```python
from build123d import *
from OCP.BRepFilletAPI import BRepFilletAPI_MakeChamfer

# Parameters (mm, degrees)
SKETCH1_W               = 27
SKETCH1_H               = 32.5
BOSS_EXTRUDE1_DEPTH     = 30
SKETCH2_W               = 14
SKETCH2_H               = 18.95
BOSS_EXTRUDE2_DEPTH     = 42.5
SKETCH3_W               = 6
SKETCH3_H               = 10
CUT_EXTRUDE1_DEPTH      = 16
FILLET1_R               = 1.49
CUT_EXTRUDE2_DEPTH      = 70.576863971
CUT_EXTRUDE2_DEPTH_BACK = 70.576863971
SKETCH4_R               = 2.1
CHAMFER1_SIZE           = 3
CHAMFER1_SIZE2          = 1.732050808
SKETCH5_W               = 5
SKETCH5_H               = 18.95
BOSS_EXTRUDE3_DEPTH     = 59
FILLET2_R               = 2


with BuildPart() as part:
    # Sketch1 → Boss-Extrude1 (new, symmetric)
    with BuildSketch(Plane.XY):
        with BuildLine():
            Line((14.75, -16.3), (14.75, 16.3))
            ThreePointArc((14.75, 16.3), (14.398528137, 17.148528137), (13.55, 17.5))
            Line((13.55, 17.5), (-13.55, 17.5))
            ThreePointArc((-13.55, 17.5), (-14.398528137, 17.148528137), (-14.75, 16.3))
            Line((-14.75, 16.3), (-14.75, -16.3))
            ThreePointArc((-14.75, -16.3), (-14.398528137, -17.148528137), (-13.55, -17.5))
            Line((-13.55, -17.5), (13.55, -17.5))
            ThreePointArc((13.55, -17.5), (14.398528137, -17.148528137), (14.75, -16.3))
        make_face()
        Rectangle(SKETCH1_W, SKETCH1_H, mode=Mode.SUBTRACT)
    extrude(amount=BOSS_EXTRUDE1_DEPTH, both=True)

    # Sketch2 → Boss-Extrude2 (add, symmetric)
    with BuildSketch(Plane(origin=(0, 0, 0), x_dir=(0, 0, -1), z_dir=(1, 0, 0))):
        with Locations((-36.5, -25.775)):
            Rectangle(SKETCH2_W, SKETCH2_H)
        with Locations((36.5, -25.775)):
            Rectangle(SKETCH2_W, SKETCH2_H)
    extrude(amount=BOSS_EXTRUDE2_DEPTH, both=True)

    # Sketch3 → Cut-Extrude1 (cut)
    with BuildSketch(Plane.XZ.offset(35.25)):
        with Locations((-27, 34.5)):
            Rectangle(SKETCH3_W, SKETCH3_H)
        with Locations((-9, 34.5)):
            Rectangle(SKETCH3_W, SKETCH3_H)
        with Locations((27, 34.5)):
            Rectangle(SKETCH3_W, SKETCH3_H)
        with Locations((9, 34.5)):
            Rectangle(SKETCH3_W, SKETCH3_H)
        with Locations((9, -34.5)):
            Rectangle(SKETCH3_W, SKETCH3_H)
        with Locations((27, -34.5)):
            Rectangle(SKETCH3_W, SKETCH3_H)
        with Locations((-9, -34.5)):
            Rectangle(SKETCH3_W, SKETCH3_H)
        with Locations((-27, -34.5)):
            Rectangle(SKETCH3_W, SKETCH3_H)
    extrude(amount=-CUT_EXTRUDE1_DEPTH, mode=Mode.SUBTRACT)

    # Fillet1
    fillet1_edges = [part.edges().sort_by_distance(p)[0] for p in [
        (6, -27.25, -39.5),
        (12, -27.25, 39.5),
        (12, -27.25, 29.5),
        (6, -27.25, 29.5),
        (6, -27.25, 39.5),
        (30, -27.25, 39.5),
        (30, -27.25, 29.5),
        (24, -27.25, 29.5),
        (24, -27.25, 39.5),
        (-12, -27.25, 29.5),
        (-12, -27.25, 39.5),
        (-6, -27.25, 39.5),
        (-6, -27.25, 29.5),
        (24, -27.25, -29.5),
        (30, -27.25, -29.5),
        (30, -27.25, -39.5),
        (24, -27.25, -39.5),
        (-12, -27.25, -29.5),
        (-6, -27.25, -29.5),
        (-6, -27.25, -39.5),
        (-12, -27.25, -39.5),
        (-30, -27.25, -29.5),
        (-24, -27.25, -29.5),
        (-24, -27.25, -39.5),
        (-30, -27.25, -39.5),
        (-30, -27.25, 29.5),
        (-30, -27.25, 39.5),
        (-24, -27.25, 39.5),
        (-24, -27.25, 29.5),
        (-42.5, -25.775, 29.5),
        (-42.5, -25.775, 43.5),
        (42.5, -25.775, 29.5),
        (42.5, -25.775, 43.5),
        (-42.5, -25.775, -29.5),
        (-42.5, -25.775, -43.5),
        (42.5, -25.775, -29.5),
        (42.5, -25.775, -43.5),
        (6, -27.25, -29.5),
        (12, -27.25, -29.5),
        (12, -27.25, -39.5),
    ]]
    fillet(fillet1_edges, radius=FILLET1_R)

    # Sketch4 → Cut-Extrude2 (cut, two sides: drawn at the far end of the back side and taken through both)
    with BuildSketch(Plane(origin=(0, -16.3, 0), x_dir=(1, 0, 0), z_dir=(0, 1, 0)).offset(-CUT_EXTRUDE2_DEPTH_BACK)):
        with Locations(Location((36.25, -36.25, 0), (0, 0, 270))):
            Circle(SKETCH4_R)
        with Locations(Location((-36.25, -36.25, 0), (0, 0, 90))):
            Circle(SKETCH4_R)
        with Locations(Location((-36.25, 36.25, 0), (0, 0, 270))):
            Circle(SKETCH4_R)
        with Locations(Location((36.25, 36.25, 0), (0, 0, 90))):
            Circle(SKETCH4_R)
    extrude(amount=CUT_EXTRUDE2_DEPTH + CUT_EXTRUDE2_DEPTH_BACK, mode=Mode.SUBTRACT)

    # Chamfer1: one chamfer whose edges measure the first distance from different faces: ONE call of the kernel's chamfer builder (chamfer() names one face for all edges)
    chamfer1_edges_1 = [part.edges().sort_by_distance(p)[0] for p in [
        (36.25, -16.3, -34.15),
        (-36.25, -16.3, -38.35),
    ]]
    chamfer1_side_1 = [part.faces().sort_by_distance(p)[0] for p in [
        (0, -16.3, -36.592952532),
    ]]
    chamfer1_edges_2 = [part.edges().sort_by_distance(p)[0] for p in [
        (-36.25, -16.3, 38.35),
        (36.25, -16.3, 34.15),
    ]]
    chamfer1_side_2 = [part.faces().sort_by_distance(p)[0] for p in [
        (0, -16.3, 36.592952532),
    ]]
    chamfer1 = BRepFilletAPI_MakeChamfer(part.part.solid().wrapped)
    for e in chamfer1_edges_1:
        chamfer1.Add(CHAMFER1_SIZE, CHAMFER1_SIZE2, e.wrapped, chamfer1_side_1[0].wrapped)  # the first distance lies on this face
    for e in chamfer1_edges_2:
        chamfer1.Add(CHAMFER1_SIZE, CHAMFER1_SIZE2, e.wrapped, chamfer1_side_2[0].wrapped)  # the first distance lies on this face
    add(Compound.cast(chamfer1.Shape()), mode=Mode.REPLACE)

    # Sketch5 → Boss-Extrude3 (add)
    with BuildSketch(Plane.XY.offset(-29.5)):
        with Locations((-36, -25.775)):
            Rectangle(SKETCH5_W, SKETCH5_H)
        with Locations((36, -25.775)):
            Rectangle(SKETCH5_W, SKETCH5_H)
    extrude(amount=BOSS_EXTRUDE3_DEPTH)

    # Fillet2
    fillet2_edges = [part.edges().sort_by_distance(p)[0] for p in [
        (-38.5, -25.775, -29.5),
        (-33.5, -25.775, -29.5),
        (-38.5, -25.775, 29.5),
        (-33.5, -25.775, 29.5),
        (33.5, -25.775, -29.5),
        (38.5, -25.775, -29.5),
        (38.5, -25.775, 29.5),
        (33.5, -25.775, 29.5),
    ]]
    fillet(fillet2_edges, radius=FILLET2_R)


solid = part.part
```
Input: part model. Units: mm. Frame: model coordinates. A direction names the side the tool comes from. Round coordinates to 2 decimals unless told otherwise and drop trailing zeros. Order: outer loops, then holes, each group sorted by start corner. A loop starts at its lowest first (then second) coordinate and runs counter-clockwise, first axis right, second up. Notation, with made-up numbers: (27.5, -26) - (53.5, -26) arc R11 cw to (53.5, -17) - close; hole circle Ø4 at (-25.5, 26). An arc over 180 degrees is marked (long way). One line per question, with ' | ' between items. Start each with the question number.
1) Ray query, probe 1 along X at (y, z) = (-26, 34); probe 2 along Z at (x, y) = (36, -26); probe 3 along Z at (x, y) = (-9.5, -29). Return the intervals inside material, ascending.
2) Cut plane A-A, the plane z = -16.5. Return the cut outline in (x, y), then the cut area to 3 significant figures.
3) Cut plane C-C, the plane z = 36.25. Give the number of separate pieces and of enclosed holes in the cut face, then the cut area to 3 significant figures.
4) Contact query for flat-ended pins moving along their axis: P1, Ø5.5, axis at y = -28, z = 13.5, coming from the +X side; P2, Ø16.5, axis at y = 4.5, z = 8.5, coming from the +X side; P3, Ø2.5, axis at x = -27, z = 32.5, coming from the -Y side; P4, Ø10, axis at x = -28.5, z = -33, coming from the -Y side. Output: stop coordinate, or through.
5) Set-up query: faces 5 (the flat face through (-38.5, -26, 0)), 6 (the cylindrical face through (-32.93, -25.64, 28.9)), 7 (the flat face through (0, -26, 29.5)). Return all of +Z, -Z, +X, -X, +Y, -Y with unobstructed straight access to the full face (end or side cutting, diameter ignored); none if empty.
6) Cut plane B-B, the plane y = 13. Return the cut outline in (x, z).
7) Cut plane D-D, the plane x = 19.5. Return the cut outline in (y, z), then the cut area to 3 significant figures.
8) Pull-direction query (X, two-part tool) for faces 1 (the cylindrical face through (-39.07, -25.64, 28.9)), 2 (the flat face through (27, -19.25, -34)), 3 (the cylindrical face through (39.1, -25.64, -28.93)), 4 (the flat face through (0, 16.25, 0)); classes: +X half, -X half, draft (parallel to the pull), parting line (faces both ways), or undercut.
Worked out:
1) probe 1: x = -42.5 to -30, -24 to -12, -6 to 6, 12 to 24, 30 to 42.5 | probe 2: z = -43.5 to -38.34, -34.16 to 34.16, 38.34 to 43.5 | probe 3: z = -43.5 to -39.5, 39.5 to 43.5
2) outline: (-38.5, -35.25) - (-33.5, -35.25) - (-33.5, -16.3) - (-38.5, -16.3) - close; (-14.75, -16.3) arc R1.2 ccw to (-13.55, -17.5) - (13.55, -17.5) arc R1.2 ccw to (14.75, -16.3) - (14.75, 16.3) arc R1.2 ccw to (13.55, 17.5) - (-13.55, 17.5) arc R1.2 ccw to (-14.75, 16.3) - close; (33.5, -35.25) - (38.5, -35.25) - (38.5, -16.3) - (33.5, -16.3) - close; hole (-13.5, -16.25) - (13.5, -16.25) - (13.5, 16.25) - (-13.5, 16.25) - close | area: 343 mm^2
3) separate pieces: 3 | enclosed holes: 0 | area: 1,060 mm^2
4) P1: stops at x = 38.5 | P2: stops at x = 14.75 | P3: stops at y = -19.25 | P4: stops at y = -35.25
5) face 5: -X, +Y, -Y | face 6: +Y, -Y | face 7: -Y
6) outline: (-14.75, -30) - (-13.5, -30) - (-13.5, 30) - (-14.75, 30) - close; (13.5, -30) - (14.75, -30) - (14.75, 30) - (13.5, 30) - close
7) outline: (-35.25, -43.5) - (-16.3, -43.5) - (-16.3, -29.5) - (-35.25, -29.5) - close; (-35.25, 29.5) - (-16.3, 29.5) - (-16.3, 43.5) - (-35.25, 43.5) - close | area: 531 mm^2
8) face 1: -X half | face 2: undercut | face 3: +X half | face 4: undercut
